The model under review builds one solid part; all positions refer to its coordinate system, in mm. A direction names the side the tool comes from. Give positions to 0.01 mm unless a question says otherwise; leave off trailing zeros. Order: outer loops, then holes, each group sorted by start corner. A loop starts at its lowest first (then second) coordinate and runs counter-clockwise, first axis right, second up. Notation, with made-up numbers: (31, 81.25) - (70, 81.25) arc R20 cw to (70, 117.25) - close; hole circle Ø2 at (42.5, -30.75). An arc over 180 degrees is marked (long way). Write item = value, one per line. Start each with the question number.
1. Machinability: for faces 4 (the flat face through (-33.042, 10.95, 17.15)), 5 (the cylindrical face through (-44.73, 19.23, 6.06)), 6 (the cylindrical face through (-4.829, 7.011, -22.265)), which of the approach directions +Z, -Z, +X, -X, +Y, -Y give a long, thin tool a straight path to every point of the face, cutting with its end or side? Answer none if there is none.
2. Wall thickness on probe 1 along X at (y, z) = (-8.5, 2.5) (3 decimals); probe 2 along Z at (x, y) = (-31, 0); probe 3 along Z at (x, y) = (-20.5, 0): over which ranges is each line inside the solid? List them lowest first.
3. For P1, Ø6, axis at x = -15, y = -9.5, coming from the -Z side; P2, Ø6, axis at x = -15, z = -4, coming from the +Y side; P3, Ø2, axis at x = -20.5, z = 10, coming from the +Y side; P4, Ø2, axis at y = -18, z = 18, coming from the -X side, all flat-tipped, find the tip position at first contact; note any pin that passes through.
4. We need section C-C, the plane x = -42.5. Give the boundary of the cut face in (y, z) (1 decimal), and give its area (3 significant figures).
5. Mouldability with a two-part tool opening along Z and no side actions: class faces 1 (the cylindrical face through (-28.308, -14.274, 0.628)), 2 (the conical face through (-21.973, 19.427, 6.118)), 3 (the flat face through (-24.332, 10.95, 17.15)) as pulls with the +Z half, pulls with the -Z half, needs draft (parallel to the pull), parting line crosses it, or undercut.
6. We need section A-A, the plane y = 0. Give the boundary of the cut face in (x, z) (1 decimal), and give its area (3 significant figures).
7. We need section D-D, the plane x = -5. Give the boundary of the cut face in (y, z), and give its area (3 significant figures).
from build123d import *

# Parameters (mm, degrees)
SKETCH2_R           = 23.3426
BOSS_EXTRUDE1_DEPTH = 9.525


with BuildPart() as part:
    # Sketch1 → Revolve1 (revolve)
    with BuildSketch(Plane.XY):
        Polygon((-47.625, 14.2875), (-9.525, 14.2875), (-9.525, 20.16125), (-6.912450581, 20.16125), (-6.912450581, 20.92325), (-15.622150436, 20.16125), (-15.622150436, 20.92325), (-24.331850291, 20.16125), (-24.331850291, 20.92325), (-33.041550145, 20.16125), (-33.041550145, 20.92325), (-41.75125, 20.16125), (-47.625, 20.16125), align=None)
    revolve(axis=Axis((-47.625, 0, 0), (1, 0, 0)))

    # Sketch2 → Boss-Extrude1 (add)
    with BuildSketch(Plane(origin=(-9.525, 0, 0), x_dir=(0, 0, -1), z_dir=(1, 0, 0))):
        Circle(SKETCH2_R)
    extrude(amount=BOSS_EXTRUDE1_DEPTH)


solid = part.part
Model answer:
q1.face_4 = none
q1.face_5 = -X
q1.face_6 = +X, -X
q2.probe_1 = -9.525 to 0
q2.probe_2 = -20.34 to -14.29, 14.29 to 20.34
q2.probe_3 = -20.5 to -14.29, 14.29 to 20.5
q3.P1 = -19.87
q3.P2 = 20.9
q3.P3 = 18.42
q3.P4 = through
q4.outline = circle Ø40.3 at (0, 0); hole circle Ø28.6 at (0, 0)
q4.area = 636 mm2
q5.face_1 = undercut
q5.face_2 = parting line crosses it
q5.face_3 = needs draft
q6.outline = (-47.6, -20.2) - (-41.8, -20.2) - (-33, -20.9) - (-33, -20.2) - (-24.3, -20.9) - (-24.3, -20.2) - (-15.6, -20.9) - (-15.6, -20.2) - (-9.5, -20.7) - (-9.5, -23.3) - (0, -23.3) - (0, 23.3) - (-9.5, 23.3) - (-9.5, 20.7) - (-15.6, 20.2) - (-15.6, 20.9) - (-24.3, 20.2) - (-24.3, 20.9) - (-33, 20.2) - (-33, 20.9) - (-41.8, 20.2) - (-47.6, 20.2) - (-47.6, 14.3) - (-9.5, 14.3) - (-9.5, -14.3) - (-47.6, -14.3) - close
q6.area = 915 mm2
q7.outline = circle Ø46.69 at (0, 0)
q7.area = 1,710 mm2
